For this review, take the finished solid that the model builds, in its own axes (mm). A direction names the side the tool comes from. Give positions to 0.01 mm unless a question says otherwise; leave off trailing zeros. Loops run counter-clockwise (first coordinate to the right, second up) from the corner with the lowest first, then second, coordinate; pieces in that order, holes last. Notation, with made-up numbers: (-14.75, -8) - (30.25, -8) arc R27 cw to (30.25, 26) - close; hole circle Ø8 at (71, 57). An arc over 180 degrees is marked (long way). Answer as CSV lines item,"result".
Autodesk Inventor part; units mm, degrees
ref_plane "YZ Plane" through (0, 0, 0) normal (1, 0, 0) x (0, 1, 0)
ref_plane "XZ Plane" through (0, 0, 0) normal (0, 1, 0) x (-1, 0, 0)
ref_plane "XY Plane" through (0, 0, 0) normal (0, 0, 1) x (1, 0, 0)
sketch "Esquisse1" plane through (0, 0, 0) normal (0, 0, 1) x (1, 0, 0)
  point P0 (0, 0)
sketch "Esquisse2" plane through (0, 0, 0) normal (0, 0, 1) x (1, 0, 0)
  line L0 (0, 2.5) -> (14.5, 2.5)
  line L1 (14.5, 2.5) -> (20, 0)
  line L2 (20, 0) -> (0, 0)
  line L3 (0, 0) -> (0, 2.5)
  dimension "d0" = 20
  dimension "d1" = 14.5
  dimension "d2" = 2.5
revolve "Révolution1" add sketch "Esquisse2" angle 360 about axis through (0, 0, 0) along (0, 1, 0)
sketch "Esquisse3" plane through (0, 0, 0) normal (0, 0, 1) x (1, 0, 0)
  line L0 (-14.5, 2.5) -> (14.5, 2.5)
  line L1 (0, 2.5) -> (14.5, 2.5)
  line L2 (14.5, 2.5) -> (14.5, 3.5)
  line L3 (14.5, 3.5) -> (0, 3.5)
  line L4 (0, 3.5) -> (0, 2.5)
  point P0 (0, 0)
  dimension "d4" = 1
  dimension "d5" = 14.5
revolve "Révolution2" add sketch "Esquisse3" angle 360 about axis through (0, 3.5, 0) along (0, -1, 0)
sketch "Esquisse4" plane through (0, 0, 0) normal (0, 0, 1) x (1, 0, 0)
  line L0 (-14.5, 3.5) -> (14.5, 3.5)
  line L1 (0, 3.5) -> (0, 6)
  line L2 (0, 6) -> (20, 6)
  line L3 (20, 6) -> (14.5, 3.5)
  line L4 (14.5, 3.5) -> (0, 3.5)
  point P0 (0, 0)
  dimension "d7" = 20
  dimension "d8" = 2.5
revolve "Révolution3" add sketch "Esquisse4" angle 360 about axis through (0, 3.5, 0) along (0, 1, 0)
sketch "Esquisse5" plane through (0, 6, 0) normal (0, 1, 0) x (1, 0, 0)
  circle A0 centre (0, 0) radius 5
  dimension "d10" = 10
extrude "Extrusion1" cut sketch "Esquisse5" against normal blind 6
properties part number "Wrist polley" material "Plastique ABS"
1) Consider section A-A on z = 0. Write out the cut boundary in (x, y).
From the geometry:
outline,"(-20, 0) - (-5, 0) - (-5, 6) - (-20, 6) - (-14.5, 3.5) - (-14.5, 2.5) - close; (5, 0) - (20, 0) - (14.5, 2.5) - (14.5, 3.5) - (20, 6) - (5, 6) - close"
2) Wall thickness on line 1 (X direction, y = 3.05, z = 0); line 2 (Z direction, x = 0, y = 2.2): over which ranges is each line inside the solid? List them lowest first. Write a range as from..to.
From the geometry:
line 1,"x = -14.5..-5, 5..14.5"
line 2,"z = -15.16..-5, 5..15.16"
3) Consider section B-B on x = 0. Write out the cut boundary in (y, z), and give its area (4 significant figures).
From the geometry:
outline,"(0, -20) - (2.5, -14.5) - (3.5, -14.5) - (6, -20) - (6, -5) - (0, -5) - close; (0, 5) - (6, 5) - (6, 20) - (3.5, 14.5) - (2.5, 14.5) - (0, 20) - close"
area,"141.5 mm^2"
4) Machinability: for faces 5 (the cylindrical face through (-1.08, 3.04, 4.88)), 6 (the conical face through (-3.218, 3.656, 14.491)), which of the approach directions +Z, -Z, +X, -X, +Y, -Y give a long, thin tool a straight path to every point of the face, cutting with its end or side? Answer none if there is none.
From the geometry:
face 5,"+Y, -Y"
face 6,"none"
5) Insertion check: P1, Ø6, axis at x = 0, z = 0, coming from the +Y side; P2, Ø2, axis at y = 0.5, z = -5, coming from the -X side. Each pin has a flat end and moves straight along its axis. Give the tip position at first contact, or say it passes through.
From the geometry:
P1,"passes through"
P2,"stops at x = -19.57"
6) Consider section C-C on y = 1.75. Write out the cut boundary in (x, z), and give its area (3 significant figures).
From the geometry:
outline,"circle Ø32.3 at (0, 0); hole circle Ø10 at (0, 0)"
area,"741 mm^2"
7) Draft analysis for pull direction Y (two halves, no side actions). For faces 1 (the flat face through (4, 0, 4)), 2 (the flat face through (4, 6, 4)), 3 (the cylindrical face through (6.691, 3.007, 12.864)), 4 (the conical face through (14.159, 2.344, 4.459)), state which applies: pulls with the +Y half, pulls with the -Y half, needs draft (parallel to the pull), parting line crosses it, or undercut.
From the geometry:
face 1,"pulls with the -Y half"
face 2,"pulls with the +Y half"
face 3,"undercut"
face 4,"undercut"
